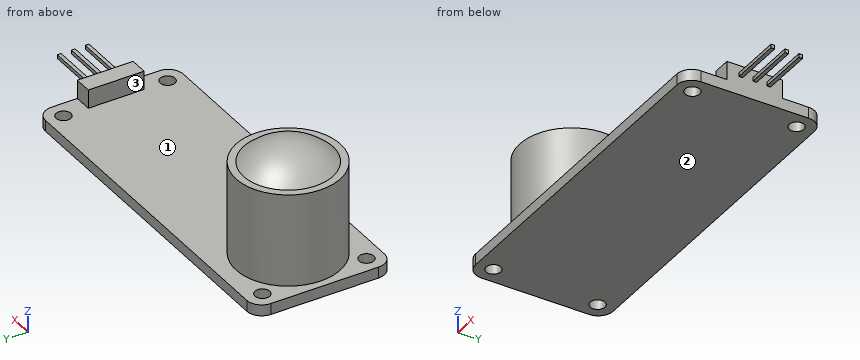
```python
from build123d import *

# Parameters (mm, degrees)
SKETCH1_W           = 48
SKETCH1_H           = 18.5
SKETCH1_R           = 1
BOSS_EXTRUDE1_DEPTH = 1.5
FILLET1_R           = 2
SKETCH2_R           = 7
BOSS_EXTRUDE2_DEPTH = 12.5
SKETCH5_W           = 2.4
SKETCH5_H           = 7.5
BOSS_EXTRUDE3_DEPTH = 2.5
SKETCH6_W           = 0.5
SKETCH6_H           = 0.5
BOSS_EXTRUDE4_DEPTH = 7


with BuildPart() as part:
    # Sketch1 → Boss-Extrude1 (new body)
    with BuildSketch(Plane.XY):
        Rectangle(SKETCH1_W, SKETCH1_H)
        with Locations((-21.75, 7)):
            Circle(SKETCH1_R, mode=Mode.SUBTRACT)
        with Locations((21.75, 7)):
            Circle(SKETCH1_R, mode=Mode.SUBTRACT)
        with Locations((21.75, -7)):
            Circle(SKETCH1_R, mode=Mode.SUBTRACT)
        with Locations((-21.75, -7)):
            Circle(SKETCH1_R, mode=Mode.SUBTRACT)
    extrude(amount=BOSS_EXTRUDE1_DEPTH)

    # Fillet1
    fillet1_edges = [part.edges().sort_by_distance(p)[0] for p in [
        (24, -9.25, 0.75),
        (-24, -9.25, 0.75),
        (-24, 9.25, 0.75),
        (24, 9.25, 0.75),
    ]]
    fillet(fillet1_edges, radius=FILLET1_R)

    # Sketch2 → Boss-Extrude2 (add)
    with BuildSketch(Plane.XY.offset(1.5)):
        with Locations(Location((-16, 0, 0), (0, 0, 180))):
            Circle(SKETCH2_R)
    extrude(amount=BOSS_EXTRUDE2_DEPTH)

    # Sketch3 → Revolve3 (revolve)
    with BuildSketch(Plane(origin=(0, 0, 0), x_dir=(-1, 0, 0), z_dir=(0, -1, 0))):
        with BuildLine():
            Line((16, -14), (16, -16.5))
            ThreePointArc((16, -16.5), (19.25, -15.85), (22, -14))
            Line((22, -14), (16, -14))
        make_face()
    revolve(axis=Axis((-16, 0, 1014), (0, 0, -1)))

    # Sketch5 → Boss-Extrude3 (add)
    with BuildSketch(Plane.XY.offset(1.5)):
        with Locations((22.8, 0)):
            Rectangle(SKETCH5_W, SKETCH5_H)
    extrude(amount=BOSS_EXTRUDE3_DEPTH)

    # Sketch6 → Boss-Extrude4 (add)
    with BuildSketch(Plane(origin=(24, 0, 0), x_dir=(0, 0, -1), z_dir=(1, 0, 0))):
        with Locations((-2.75, 1.875)):
            Rectangle(SKETCH6_W, SKETCH6_H)
        with Locations((-2.75, 0)):
            Rectangle(SKETCH6_W, SKETCH6_H)
        with Locations((-2.75, -1.875)):
            Rectangle(SKETCH6_W, SKETCH6_H)
    extrude(amount=BOSS_EXTRUDE4_DEPTH)


solid = part.part
```
The model under review builds one solid part; all positions refer to its coordinate system, in mm. Face numbers are marked on the shaded views. Round coordinates to 2 decimals unless told otherwise and drop trailing zeros. Loops run counter-clockwise (first coordinate to the right, second up) from the corner with the lowest first, then second, coordinate; pieces in that order, holes last. Notation, with made-up numbers: (86.5, -5.75) -> (142.5, -5.75) arc R29 ccw to (142.5, 32.25) -> close; hole circle Ø6 at (57, -14.5). An arc over 180 degrees is marked (long way). Answer as a JSON object with one key per item and string values. Group by question number.
1) For pin 1 Ø6 at (y, z) = (2.5, 10) entering from -X; pin 2 Ø1 at (x, y) = (-4, -6.5) entering from +Z; pin 3 Ø2 at (y, z) = (2.5, 1.5) entering from +X, all flat-tipped, find the tip position at first contact; note any pin that passes through.
2) We need section C-C on z = 10.5. Write out the cut boundary in (x, y).
3) Mouldability with a two-part tool opening along X and no side actions: class the marked faces 1, 2 and 3 as released by +X, released by -X, zero draft, split by the parting line, or undercut.
4) For line 1 (Y direction, x = -21.75, z = 0.8); line 2 (Z direction, x = 10.5, y = -7.25); line 3 (X direction, y = 4.5, z = 5.5), list the stretches that pass through material, from the lowest coordinate up. Write a range as [from, to].
5) We need section A-A on x = -16. Write out the cut boundary in (y, z).
6) We need section B-B on y = 3.25. Write out the cut boundary in (x, z).
Result set:
{
 "1": {"pin 1": "x = -23", "pin 2": "z = 1.5", "pin 3": "x = 24"},
 "2": {"outline": "circle Ø14 at (-16, 0)"},
 "3": {"face 1": "undercut", "face 2": "zero draft", "face 3": "undercut"},
 "4": {"line 1": "[-9.25, -8], [-6, 6], [8, 9.25]", "line 2": "[0, 1.5]", "line 3": "[-21.36, -10.64]"},
 "5": {"outline": "(-9.25, 0) -> (9.25, 0) -> (9.25, 1.5) -> (7, 1.5) -> (7, 14) -> (6, 14) arc R8.45 ccw to (-6, 14) -> (-7, 14) -> (-7, 1.5) -> (-9.25, 1.5) -> close"},
 "6": {"outline": "(-24, 0) -> (24, 0) -> (24, 4) -> (21.6, 4) -> (21.6, 1.5) -> (-9.8, 1.5) -> (-9.8, 14) -> (-10.96, 14) arc R7.8 ccw to (-21.04, 14) -> (-22.2, 14) -> (-22.2, 1.5) -> (-24, 1.5) -> close"}
}
